Read the model definition and answer for the solid it produces. Units are mm, in the model's axes. A direction names the side the tool comes from. Give positions to 0.01 mm unless a question says otherwise; leave off trailing zeros. Write each loop counter-clockwise with the first axis right and the second up, starting at its lowest first coordinate (ties: lowest second). Pieces come first, ordered by that corner, then holes. Notation, with made-up numbers: M 64.5,31 L 96.5,31 A15 ccw 96.5,36 Z; hole C 23.25,73 d1. An arc over 180 degrees is marked long. Use a Markdown table: item, result. Add a question column.
Item 1: A cutting plane is placed at B-B on x = -44. Determine the outline of the cut face in (y, z).
Item 2: The mould has two halves that part along X. Classify faces 4 (the flat face through (-8, -130, 2)), 5 (the flat face through (-45, -135, 3)), 6 (the flat face through (-15, 7, 3)), 7 (the flat face through (-90, -113, 2)): pulls with the +X half, pulls with the -X half, needs draft (parallel to the pull), parting line crosses it, or undercut.
Item 3: Consider probe 1 along Y at (x, z) = (-50.5, 2.5); probe 2 along X at (y, z) = (-63, 2.3); probe 3 along Y at (x, z) = (3, 3.95). Determine where each line is inside the solid, lowest interval first. Write a range as [from, to].
Item 4: Given P1, Ø1.5, axis at y = 7, z = 2, coming from the -X side; P2, Ø2.5, axis at x = 2.5, z = 3.5, coming from the +Y side; P3, Ø1.5, axis at x = -80.5, z = 2.5, coming from the -Y side, each flat-ended and moving along its own axis, determine where each tip first touches the part or whether it passes through.
Item 5: A cutting plane is placed at C-C on z = 3.15. Count the separate pieces of the cut face and the enclosed holes in it, then the cut area to 3 significant figures.
Item 6: A cutting plane is placed at D-D on x = -13. Determine the outline of the cut face in (y, z), then the cut area to 3 significant figures.
Item 7: A cutting plane is placed at A-A on y = -62. Determine the outline of the cut face in (x, z).
Item 8: For faces 1 (the flat face through (-97, -95, 2)), 2 (the flat face through (-20, 7, 3)), 3 (the flat face through (-15, -135, 3)), determine the directions among +Z, -Z, +X, -X, +Y, -Y from which every point of the face is accessible in a straight line to the end or side of a thin tool.
from build123d import *

# Parameters (mm, degrees)
SKETCH1_W           = 90
SKETCH1_H           = 130
BOSS_EXTRUDE1_DEPTH = 5
SKETCH2_W           = 60
SKETCH2_H           = 15
SKETCH2_W_2         = 50
SKETCH2_H_2         = 5
BOSS_EXTRUDE2_DEPTH = 5
SKETCH3_W           = 50
SKETCH3_H           = 5
BOSS_EXTRUDE3_DEPTH = 5
SKETCH4_W           = 15
SKETCH4_H           = 60
SKETCH4_W_2         = 5
SKETCH4_H_2         = 50
BOSS_EXTRUDE4_DEPTH = 5


with BuildPart() as part:
    # Sketch1 → Boss-Extrude1 (new body)
    with BuildSketch(Plane.XY):
        with Locations((-45, -65)):
            Rectangle(SKETCH1_W, SKETCH1_H)
    extrude(amount=BOSS_EXTRUDE1_DEPTH)

    # Sketch2 → Boss-Extrude2 (add)
    # profile 1 of 2: a face of its own
    with BuildSketch(Plane.XY.offset(5)):
        with Locations((-45, 7.5)):
            Rectangle(SKETCH2_W, SKETCH2_H)
        with Locations((-45, 7.5)):
            Rectangle(SKETCH2_W_2, SKETCH2_H_2, mode=Mode.SUBTRACT)
    # profile 2 of 2: a face of its own
    with BuildSketch(Plane.XY.offset(5)):
        Polygon((-15, -140), (-15, -130), (-20, -130), (-20, -135), (-70, -135), (-70, -130), (-75, -130), (-75, -140), align=None)
    extrude(amount=-BOSS_EXTRUDE2_DEPTH)

    # Sketch3 → Boss-Extrude3 (add)
    # profile 1 of 2: a face of its own
    with BuildSketch(Plane.XY.offset(5)):
        Polygon((0, -130), (0, -95), (0, -90), (0, -40), (0, -35), (0, 0), (-15, 0), (-15, 15), (-75, 15), (-75, 0), (-90, 0), (-90, -130), (-75, -130), (-75, -140), (-15, -140), (-15, -130), align=None)
        with Locations((-45, -132.5)):
            Rectangle(SKETCH3_W, SKETCH3_H, mode=Mode.SUBTRACT)
        with Locations((-45, 7.5)):
            Rectangle(SKETCH3_W, SKETCH3_H, mode=Mode.SUBTRACT)
    # profile 2 of 2: a face of its own
    with BuildSketch(Plane.XY.offset(5)):
        Polygon((0, -95), (10, -95), (10, -35), (0, -35), (0, -40), (5, -40), (5, -90), (0, -90), align=None)
    extrude(amount=-BOSS_EXTRUDE3_DEPTH)

    # Sketch4 → Boss-Extrude4 (add)
    with BuildSketch(Plane(origin=(0, 0, 0), x_dir=(-1, 0, 0), z_dir=(0, 0, -1))):
        with Locations((97.5, -65)):
            Rectangle(SKETCH4_W, SKETCH4_H)
        with Locations((97.5, -65)):
            Rectangle(SKETCH4_W_2, SKETCH4_H_2, mode=Mode.SUBTRACT)
    extrude(amount=-BOSS_EXTRUDE4_DEPTH)


solid = part.part
Filled in:
| question | item | result |
|---|---|---|
| 1 | outline | M -140,0 L -135,0 L -135,5 L -140,5 Z; M -130,0 L 5,0 L 5,5 L -130,5 Z; M 10,0 L 15,0 L 15,5 L 10,5 Z |
| 2 | face 4 | needs draft |
| 2 | face 5 | undercut |
| 2 | face 6 | pulls with the +X half |
| 2 | face 7 | pulls with the -X half |
| 3 | probe 1 | [-140, -135], [-130, 5], [10, 15] |
| 3 | probe 2 | [-105, -100], [-95, 0], [5, 10] |
| 3 | probe 3 | [-95, -90], [-40, -35] |
| 4 | P1 | x = -75 |
| 4 | P2 | y = -35 |
| 4 | P3 | y = -130 |
| 5 | separate pieces | 1 |
| 5 | enclosed holes | 4 |
| 5 | area | 13,700 mm² |
| 6 | outline | M -130,0 L 0,0 L 0,5 L -130,5 Z |
| 6 | area | 650 mm² |
| 7 | outline | M -105,0 L -100,0 L -100,5 L -105,5 Z; M -95,0 L 0,0 L 0,5 L -95,5 Z; M 5,0 L 10,0 L 10,5 L 5,5 Z |
| 8 | face 1 | +Z, -Z, -X, -Y |
| 8 | face 2 | +Z, -Z |
| 8 | face 3 | +Z, -Z, +X, -Y |
